Build history of the part. All positions in model axes, mm. A direction names the side the tool comes from. Give positions to 0.01 mm unless a question says otherwise; leave off trailing zeros. Loops run counter-clockwise (first coordinate to the right, second up) from the corner with the lowest first, then second, coordinate; pieces in that order, holes last. Notation, with made-up numbers: M 3,-34.75 L 58,-34.75 A18 cw 58,-21.75 Z; hole C 88,-29 d1. An arc over 180 degrees is marked long. Put each result on its own line as item: value.
```python
from build123d import *

# Parameters (mm, degrees)
F2_W = 0.2
F2_H = 0.2


with BuildPart() as f1:
    # F0 (on Right) → F1 (revolve)
    with BuildSketch(Plane.YZ):
        Polygon((-0.8, 0.5), (-0.8, 0), (7.9, 0), (7.9, 0.5), (5.4, 0.5), (5.4, 1.2), (3.9, 1.2), (3.9, 0.5), (3, 0.5), (3, 1.4), (0, 1.4), (0, 0.5), align=None)
    revolve(axis=Axis((0, 3.55, 0), (0, -1, 0)))

    # F2 (on Right) → F3 (revolve, cut)
    with BuildSketch(Plane.YZ):
        with Locations((2.9, 1.3)):
            Rectangle(F2_W, F2_H)
        with Locations((0.1, 1.3)):
            Rectangle(F2_W, F2_H)
    revolve(axis=Axis((0, 1.5, 0), (0, 1, 0)), mode=Mode.SUBTRACT)

    # F4 (on Right) → F5 (revolve)
    with BuildSketch(Plane.YZ):
        Polygon((4, 1.4), (4, 1.2), (4.9, 1.2), (5.3, 1.2), (5.3, 1.4), align=None)
    revolve(axis=Axis((0, 4.65, 0), (0, 1, 0)))


solid = f1.part
```
Q1. Drop a flat-ended pin along its axis: pin 1 Ø1 at (x, z) = (-0.5, 1) entering from +Y. Give the stop position or say it passes through.
Here are the results:
pin 1: y = 5.4
Q2. Slice it at B-B (x = -0.9). List the corners of the cut face in (y, z).
Here are the results:
outline: M 0,-0.79 L 0.2,-0.79 L 0.2,-1.07 L 2.8,-1.07 L 2.8,-0.79 L 3,-0.79 L 3,0.79 L 2.8,0.79 L 2.8,1.07 L 0.2,1.07 L 0.2,0.79 L 0,0.79 Z; M 3.9,-0.79 L 4,-0.79 L 4,-1.07 L 5.3,-1.07 L 5.3,-0.79 L 5.4,-0.79 L 5.4,0.79 L 5.3,0.79 L 5.3,1.07 L 4,1.07 L 4,0.79 L 3.9,0.79 Z
Q3. Tool access for faces 5 (the flat face through (1, 0, 0)), 6 (the flat face through (1, 3.9, 0)), 7 (the cylindrical face through (0.06, 4.64, -1.4)): list every direction of +Z, -Z, +X, -X, +Y, -Y with a clear straight run to the whole face (end or side of a thin tool).
Here are the results:
face 5: -Y
face 6: none
face 7: +Y, -Y
Q4. Probe line 1 (Y direction, x = -0.55, z = -0.15); line 2 (Y direction, x = -1.15, z = -0.75); line 3 (X direction, y = 0.25, z = -0.65). List the from-to ranges inside material, lowest first. Write a range as from..to.
Here are the results:
line 1: 0..3, 3.9..5.4
line 2: 0.2..2.8, 4..5.3
line 3: -1.24..1.24
Q5. Slice it at C-C (y = 6). List the corners of the cut face in (x, z).
Here are the results:
outline: C 0,0 d1
Q6. Slice it at A-A (z = -0.7). List the corners of the cut face in (x, y).
Here are the results:
outline: M -1.21,0.2 L -0.97,0.2 L -0.97,0 L 0.97,0 L 0.97,0.2 L 1.21,0.2 L 1.21,2.8 L 0.97,2.8 L 0.97,3 L -0.97,3 L -0.97,2.8 L -1.21,2.8 Z; M -1.21,4 L -0.97,4 L -0.97,3.9 L 0.97,3.9 L 0.97,4 L 1.21,4 L 1.21,5.3 L 0.97,5.3 L 0.97,5.4 L -0.97,5.4 L -0.97,5.3 L -1.21,5.3 Z
Q7. Mould opens along Y. For faces 1 (the flat face through (1, 5.4, 0)), 2 (the cylindrical face through (0.488, 6.632, -0.108)), 3 (the flat face through (1, 3, 0)), 4 (the cylindrical face through (0.488, 3.444, -0.108)) say: pulls with the +Y half, pulls with the -Y half, needs draft (parallel to the pull), parting line crosses it, or undercut.
Here are the results:
face 1: pulls with the +Y half
face 2: needs draft
face 3: undercut
face 4: undercut
